from build123d import *

# Parameters (mm, degrees)
SKETCH1_R                 = 7.5
BOSS_EXTRUDE1_DEPTH       = 37
SKETCH2_W                 = 3.5
SKETCH2_H                 = 29
CUT_EXTRUDE1_DEPTH        = 6
CUT_EXTRUDE2_DEPTH        = 6
SKETCH6_R                 = 5
CUT_EXTRUDE3_DEPTH        = 5
SKETCH10_OUTSIDE_W        = 25.53
SKETCH10_OUTSIDE_H        = 25.53
SKETCH10_OUTSIDE_W_2      = 6
SKETCH10_OUTSIDE_H_2      = 6
CUT_EXTRUDE4_DEPTH        = 3
SKETCH19_R                = 4.909942114
SKETCH19_R_2              = 3.5
CUT_EXTRUDE5_DEPTH        = 4
M4X0_7_TAPPED_HOLE1_D     = 3.3
M4X0_7_TAPPED_HOLE1_DEPTH = 10.1
M4X0_7_TAPPED_HOLE1_TIP   = 0.991420021
SKETCH17_W                = 0.75
SKETCH17_H                = 2
CHAMFER1_SIZE             = 0.2
CHAMFER2_SIZE             = 0.2


with BuildPart() as part:
    # Sketch1 → Boss-Extrude1 (new body)
    with BuildSketch(Plane.XY):
        Circle(SKETCH1_R)
    extrude(amount=-BOSS_EXTRUDE1_DEPTH)

    # Sketch2 → Cut-Revolve1 (revolve, cut)
    with BuildSketch(Plane(origin=(0, 0, 0), x_dir=(1, 0, 0), z_dir=(0, 1, 0))):
        with Locations((5.75, 22.5)):
            Rectangle(SKETCH2_W, SKETCH2_H)
    revolve(axis=Axis((0, 0, 0), (0, 0, -1)), mode=Mode.SUBTRACT)

    # Sketch4 → Cut-Extrude1 (cut)
    with BuildSketch(Plane.XY):
        with BuildLine():
            Line((-9.646529656, 1), (9.646529656, 1))
            ThreePointArc((9.646529656, 1), (10.646529656, 0), (9.646529656, -1))
            Line((9.646529656, -1), (-9.646529656, -1))
            ThreePointArc((-9.646529656, -1), (-10.646529656, 0), (-9.646529656, 1))
        make_face()
    extrude(amount=-CUT_EXTRUDE1_DEPTH, mode=Mode.SUBTRACT)

    # Sketch5 → Cut-Extrude2 (cut)
    with BuildSketch(Plane.XY):
        with BuildLine():
            Line((1, 8.5), (1, -8.5))
            ThreePointArc((1, -8.5), (0, -9.5), (-1, -8.5))
            Line((-1, -8.5), (-1, 8.5))
            ThreePointArc((-1, 8.5), (0, 9.5), (1, 8.5))
        make_face()
    extrude(amount=-CUT_EXTRUDE2_DEPTH, mode=Mode.SUBTRACT)

    # Sketch6 → Cut-Extrude3 (cut)
    with BuildSketch(Plane.XY):
        Circle(SKETCH6_R)
    extrude(amount=-CUT_EXTRUDE3_DEPTH, mode=Mode.SUBTRACT)

    # Sketch10 outside → Cut-Extrude4 (cut)
    with BuildSketch(Plane(origin=(0, 0, -37), x_dir=(-1, 0, 0), z_dir=(0, 0, -1))):
        Rectangle(SKETCH10_OUTSIDE_W, SKETCH10_OUTSIDE_H)
        Rectangle(SKETCH10_OUTSIDE_W_2, SKETCH10_OUTSIDE_H_2, mode=Mode.SUBTRACT)
    extrude(amount=-CUT_EXTRUDE4_DEPTH, mode=Mode.SUBTRACT)

    # Sketch19 → Cut-Extrude5 (cut, through all)
    with BuildSketch(Plane(origin=(0, 0, -34), x_dir=(-1, 0, 0), z_dir=(0, 0, -1))):
        Circle(SKETCH19_R)
        Circle(SKETCH19_R_2, mode=Mode.SUBTRACT)
    extrude(amount=CUT_EXTRUDE5_DEPTH, mode=Mode.SUBTRACT)

    # M4x0.7 Tapped Hole1
    with Locations(Plane(origin=(0, 0, -37), x_dir=(-1, 0, 0), z_dir=(0, 0, -1))):
        with Locations((0, 0)):
            Hole(M4X0_7_TAPPED_HOLE1_D / 2, depth=M4X0_7_TAPPED_HOLE1_DEPTH)
            with Locations((0, 0, -(M4X0_7_TAPPED_HOLE1_DEPTH + M4X0_7_TAPPED_HOLE1_TIP / 2))):  # 118° drill point
                Cone(0, M4X0_7_TAPPED_HOLE1_D / 2, M4X0_7_TAPPED_HOLE1_TIP, mode=Mode.SUBTRACT)

    # Sketch17 → Revolve1 (revolve)
    with BuildSketch(Plane(origin=(0, 0, 0), x_dir=(1, 0, 0), z_dir=(0, 1, 0))):
        with Locations((4.375, 13)):
            Rectangle(SKETCH17_W, SKETCH17_H)
    revolve(axis=Axis((0, 0, 0), (0, 0, -1)))

    # Chamfer1
    chamfer1_edges = [part.edges().sort_by_distance(p)[0] for p in [
        (-4.75, 0, -12),
        (-4.75, 0, -14),
    ]]
    chamfer(chamfer1_edges, length=CHAMFER1_SIZE)

    # Chamfer2
    chamfer2_edges = [part.edges().sort_by_distance(p)[0] for p in [
        (-5.303300859, -5.303300859, 0),
        (5.303300859, 5.303300859, 0),
        (5.303300859, -5.303300859, 0),
        (-5.303300859, 5.303300859, 0),
        (-7.5, 0, -8),
        (-3.535533906, -3.535533906, 0),
        (3.535533906, -3.535533906, 0),
        (3.535533906, 3.535533906, 0),
        (-3.535533906, 3.535533906, 0),
    ]]
    chamfer(chamfer2_edges, length=CHAMFER2_SIZE)


solid = part.part
For this review, take the finished solid that the model builds, in its own axes (mm). A direction names the side the tool comes from. Give positions to 0.01 mm unless a question says otherwise; leave off trailing zeros. Loops run counter-clockwise (first coordinate to the right, second up) from the corner with the lowest first, then second, coordinate; pieces in that order, holes last.
Item 1: Take a section at B-B, the plane z = -14.5. State the section outline as (x, y) points, and give its area (3 significant figures).
Item 2: Tool access review of faces 1 (the cylindrical face through (-3.51, 3.56, -2.57)), 2 (the cylindrical face through (2.47, 2.48, -35.48)), 3 (the flat face through (1, -6, -4)), 4 (the cylindrical face through (2.48, -2.47, -35.48)), 5 (the flat face through (-3, 3, -12)): name each direction out of +Z, -Z, +X, -X, +Y, -Y from which nothing blocks a thin tool from reaching the whole face with its end or side.
Item 3: For line 1 along Y through (x, z) = (0, -30); line 2 along Z through (x, y) = (4, 2.25), list the stretches that pass through material, from the lowest coordinate up.
Item 4: Insertion check: pin 1 (6.5 mm diameter, centred on y = -5.5, z = -4, fed in from -X); pin 2 (3 mm diameter, centred on x = -4, z = -1.5, fed in from +Y); pin 3 (1.5 mm diameter, centred on y = 0, z = -35.5, fed in from +X). Each pin has a flat end and moves straight along its axis. Give the tip position at first contact, or say it passes through.
Item 5: Draft analysis for pull direction Z (two halves, no side actions). For faces 6 (the cylindrical face through (-0.867, 3.905, -24.14)), 7 (the flat face through (-3.2, 0, -34)), 8 (the cylindrical face through (-0.867, 3.905, -10.028)), state which applies: +Z half, -Z half, draft (parallel to the pull), parting line (faces both ways), or undercut.
Item 6: Take a section at A-A, the plane z = -31.5. State the section outline as (x, y) points.
Calculated:
1. outline: circle Ø8 at (0, 0)
1. area: 50.3 mm2
2. face 1: +Z
2. face 2: -Z, +X, +Y
2. face 3: +Z, +Y, -Y
2. face 4: -Z, +X, -Y
2. face 5: none
3. line 1: y = -4 to -1.65, 1.65 to 4
3. line 2: z = -13.96 to -12.04, -8 to -5
4. pin 1: stops at x = -7.15
4. pin 2: stops at y = 7.07
4. pin 3: stops at x = 3
5. face 6: draft
5. face 7: -Z half
5. face 8: undercut
6. outline: circle Ø8 at (0, 0); hole circle Ø3.3 at (0, 0)
